Check sheet for the drawn part. Datum: minimum x, y, z corner. Units: mm. Round coordinates to 2 decimals unless told otherwise and drop trailing zeros. Write each loop counter-clockwise with the first axis right and the second up, starting at its lowest first coordinate (ties: lowest second). Pieces come first, ordered by that corner, then holes.
Item 1: Material ranges on line 1 (Y direction, x = 28.5, z = 0.5), recorded low to high.
Item 2: Cross-section at A-A on y = 9. Enter the section's corners in (x, z).
Item 3: Cross-section at C-C on x = 21. Enter the section's corners in (y, z), plus the area to 3 significant figures.
Item 4: Cross-section at B-B on z = 1.1. Enter the section's corners in (x, y), plus the area to 3 significant figures.
Item 5: Go/stop test with flat-tipped pins: pin 1 Ø0.9 at (x, z) = (23.5, 2) entering from -Y; pin 2 Ø1.5 at (y, z) = (3, 2) entering from -X; pin 3 Ø1.5 at (y, z) = (3.5, 2) entering from +X. Record where each tip stops, or that it passes through.
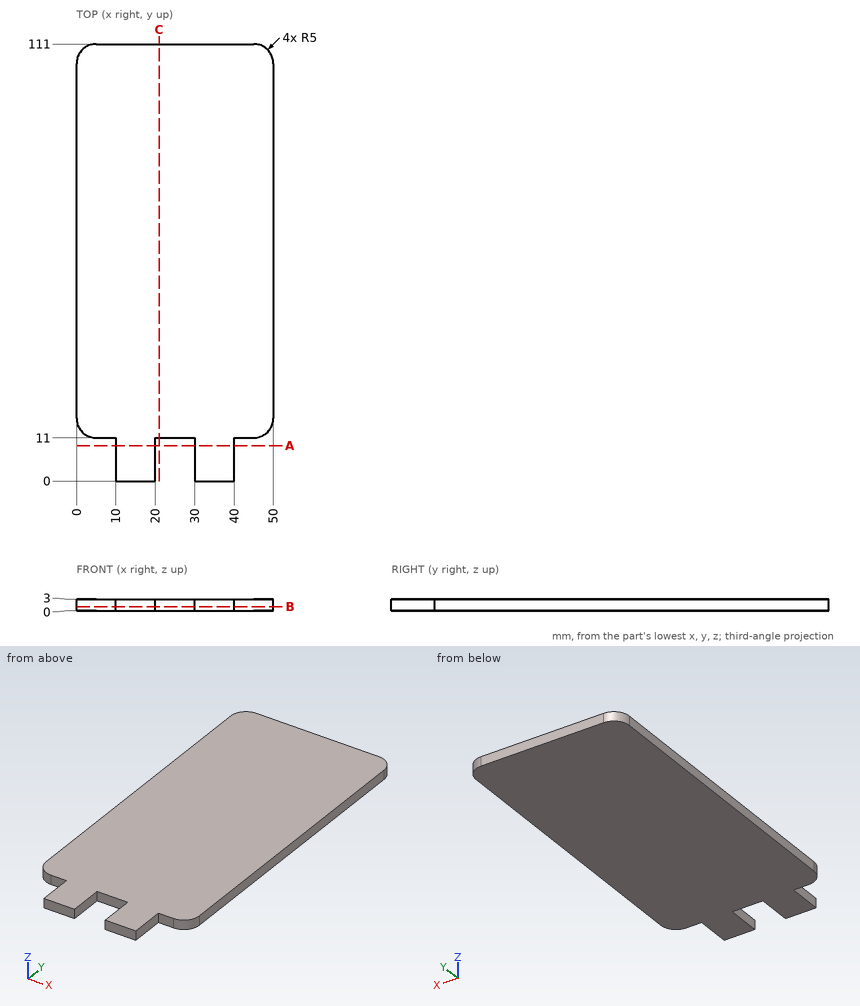
Response values:
1. line 1: y = 11 to 111
2. outline: (10, 0) - (20, 0) - (20, 3) - (10, 3) - close; (30, 0) - (40, 0) - (40, 3) - (30, 3) - close
3. outline: (11, 0) - (111, 0) - (111, 3) - (11, 3) - close
3. area: 300 mm2
4. outline: (0, 16) arc R5 ccw to (5, 11) - (10, 11) - (10, 0) - (20, 0) - (20, 11) - (30, 11) - (30, 0) - (40, 0) - (40, 11) - (45, 11) arc R5 ccw to (50, 16) - (50, 106) arc R5 ccw to (45, 111) - (5, 111) arc R5 ccw to (0, 106) - close
4. area: 5,200 mm2
5. pin 1: stops at y = 11
5. pin 2: stops at x = 10
5. pin 3: stops at x = 40
